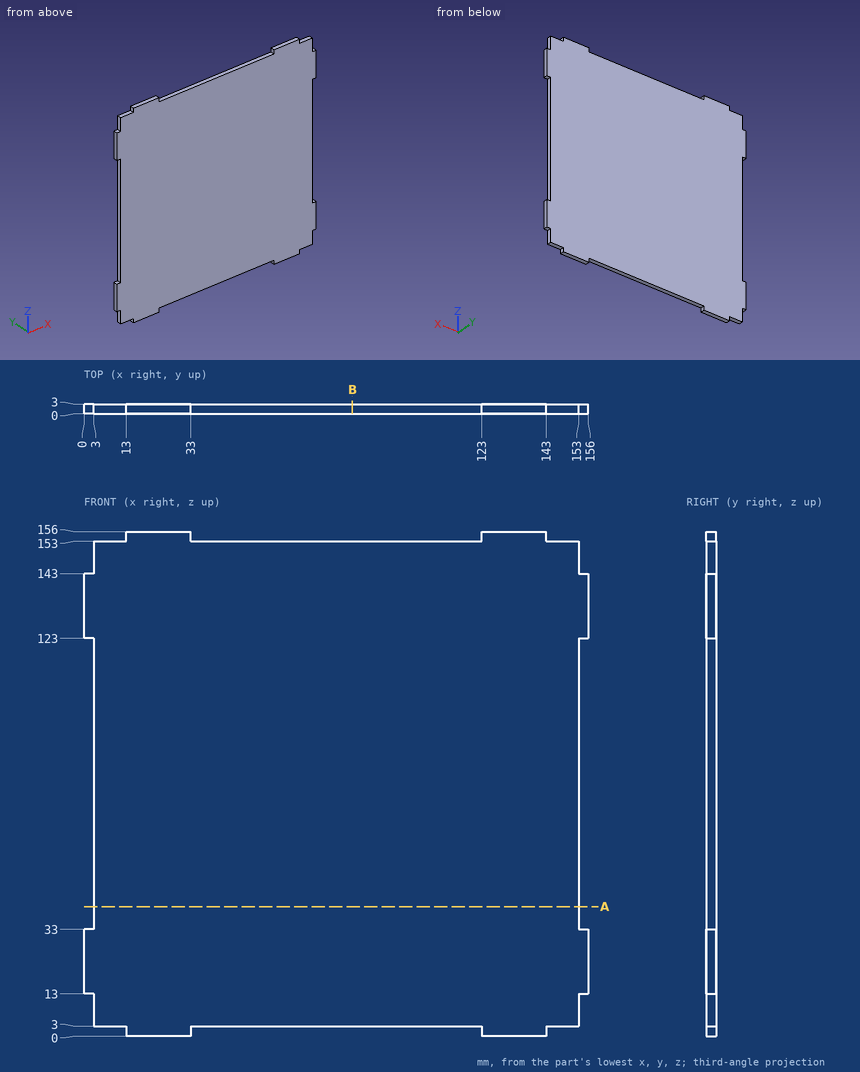
Input: dimensioned drawing with shaded views. Units: mm. Origin: part minimum x, y, z. Round coordinates to 2 decimals unless told otherwise and drop trailing zeros. Order: outer loops, then holes, each group sorted by start corner. A loop starts at its lowest first (then second) coordinate and runs counter-clockwise, first axis right, second up. Notation, with made-up numbers: (13.5, -5) - (38.5, -5) arc R28 cw to (38.5, 22) - close; hole circle Ø4 at (-34, -32.75). An arc over 180 degrees is marked (long way). Use CSV: the item, a comma, the result in double quotes. Start each with the question number.
Q1. Material intervals for line 1 along Z through (x, y) = (33.5, 2), sorted ascending. Write a range as from..to.
Q2. Section query B-B (x = 83). Return loops of the section in (y, z).
Q3. First-contact query: pin 1 (1.5 mm diameter, centred on x = 148, y = 2, fed in from -Z); pin 2 (3 mm diameter, centred on x = 62, z = 104, fed in from -Y); pin 3 (0.9 mm diameter, centred on y = 1, z = 149, fed in from -X); pin 4 (1.5 mm diameter, centred on y = 1, z = 1.5, fed in from +X). Flat tips, straight axial feed; report the tip coordinate or a pass-through.
Q4. Section query A-A (z = 40). Return loops of the section in (x, y).
Result set:
1,line 1,"z = 3..153"
2,outline,"(0, 3) - (3, 3) - (3, 153) - (0, 153) - close"
3,pin 1,"stops at z = 3"
3,pin 2,"stops at y = 0"
3,pin 3,"stops at x = 3"
3,pin 4,"stops at x = 143"
4,outline,"(3, 0) - (153, 0) - (153, 3) - (3, 3) - close"
